from build123d import *

# Parameters (mm, degrees)
SKETCH1_R           = 4.064
BOSS_EXTRUDE1_DEPTH = 56.896
SKETCH2_R           = 15.24
BOSS_EXTRUDE2_DEPTH = 25.4
SKETCH3_R           = 17.501560838
BOSS_EXTRUDE3_DEPTH = 5.588


with BuildPart() as part:
    # Sketch1 → Boss-Extrude1 (new body)
    with BuildSketch(Plane(origin=(0, 0, 0), x_dir=(1, 0, 0), z_dir=(0, 1, 0))):
        with BuildLine():
            Line((-80.173724845, 32.537607562), (-20.229724845, 32.537607562))
            ThreePointArc((-20.229724845, 32.537607562), (-16.278412152, 30.900920256), (-14.641724845, 26.949607562))
            Line((-14.641724845, 26.949607562), (-14.641724845, -32.994392438))
            ThreePointArc((-14.641724845, -32.994392438), (-16.278412152, -36.945705131), (-20.229724845, -38.582392438))
            Line((-20.229724845, -38.582392438), (-80.173724845, -38.582392438))
            ThreePointArc((-80.173724845, -38.582392438), (-84.125037539, -36.945705131), (-85.761724845, -32.994392438))
            Line((-85.761724845, -32.994392438), (-85.761724845, 26.949607562))
            ThreePointArc((-85.761724845, 26.949607562), (-84.125037539, 30.900920256), (-80.173724845, 32.537607562))
        make_face()
        with Locations((-80.173724845, 26.949607562)):
            Circle(SKETCH1_R, mode=Mode.SUBTRACT)
        with Locations((-80.173724845, -32.994392438)):
            Circle(SKETCH1_R, mode=Mode.SUBTRACT)
        with Locations((-20.229724845, 26.949607562)):
            Circle(SKETCH1_R, mode=Mode.SUBTRACT)
        with Locations((-20.229724845, -32.994392438)):
            Circle(SKETCH1_R, mode=Mode.SUBTRACT)
    extrude(amount=BOSS_EXTRUDE1_DEPTH)

    # Sketch2 → Boss-Extrude2 (add)
    with BuildSketch(Plane.XZ):
        with Locations((-50.201724845, 3.022392438)):
            Circle(SKETCH2_R)
    extrude(amount=BOSS_EXTRUDE2_DEPTH)

    # Sketch3 → Boss-Extrude3 (add)
    with BuildSketch(Plane.XZ.offset(25.4)):
        with Locations((-50.201724845, 3.022392438)):
            Circle(SKETCH3_R)
    extrude(amount=BOSS_EXTRUDE3_DEPTH)


solid = part.part
Check sheet for the modelled part. Datum: model origin and axes. Units: mm. A direction names the side the tool comes from. Give positions to 0.01 mm unless a question says otherwise; leave off trailing zeros. Order: outer loops, then holes, each group sorted by start corner. A loop starts at its lowest first (then second) coordinate and runs counter-clockwise, first axis right, second up. Notation, with made-up numbers: (-10, 21.5) - (43, 21.5) arc R9 cw to (43, 30.5) - close; hole circle Ø5 at (-21, 44.5). An arc over 180 degrees is marked (long way). Answer as CSV lines item,"result".
1. Section check D-D (z = 14.5). Record the boundary of the cut face in (x, y), then the cut area to 3 significant figures.
Result sheet:
outline,"(-85.76, 0) - (-60.23, 0) - (-60.23, -25.4) - (-63.41, -25.4) - (-63.41, -30.99) - (-36.99, -30.99) - (-36.99, -25.4) - (-40.18, -25.4) - (-40.18, 0) - (-14.64, 0) - (-14.64, 56.9) - (-85.76, 56.9) - close"
area,"4,700 mm²"
2. Section check B-B (z = -24.5). Record the boundary of the cut face in (x, y).
Result sheet:
outline,"(-85.76, 0) - (-83.42, 0) - (-83.42, 56.9) - (-85.76, 56.9) - close; (-76.93, 0) - (-23.47, 0) - (-23.47, 56.9) - (-76.93, 56.9) - close; (-16.99, 0) - (-14.64, 0) - (-14.64, 56.9) - (-16.99, 56.9) - close"
3. Section check C-C (x = -19). Record the boundary of the cut face in (y, z).
Result sheet:
outline,"(0, -32.4) - (56.9, -32.4) - (56.9, -30.82) - (0, -30.82) - close; (0, -23.08) - (56.9, -23.08) - (56.9, 29.12) - (0, 29.12) - close; (0, 36.87) - (56.9, 36.87) - (56.9, 38.45) - (0, 38.45) - close"
4. Section check A-A (y = 5.5). Record the boundary of the cut face in (x, z), then the cut area to 3 significant figures.
Result sheet:
outline,"(-85.76, -26.95) arc R5.59 ccw to (-80.17, -32.54) - (-20.23, -32.54) arc R5.59 ccw to (-14.64, -26.95) - (-14.64, 32.99) arc R5.59 ccw to (-20.23, 38.58) - (-80.17, 38.58) arc R5.59 ccw to (-85.76, 32.99) - close; hole circle Ø8.13 at (-80.17, -26.95); hole circle Ø8.13 at (-80.17, 32.99); hole circle Ø8.13 at (-20.23, -26.95); hole circle Ø8.13 at (-20.23, 32.99)"
area,"4,820 mm²"
5. Scan lines: probe 1 along Z at (x, y) = (-80.5, 48.5); probe 2 along Z at (x, y) = (-80, 41.5); probe 3 along X at (y, z) = (15.5, -25). Record each from-to range of solid material in increasing order. Write a range as from..to.
Result sheet:
probe 1,"-32.53..-31, -22.9..28.94, 37.05..38.57"
probe 2,"-32.54..-31.01, -22.89..28.93, 37.05..38.58"
probe 3,"-85.76..-83.74, -76.61..-23.8, -16.66..-14.64"
6. Tool access check on faces 1 (the face through (-51, 28, -32.538)), 2 (the face through (-34.035, -28.155, -3.681)), 3 (the face through (-65.427, -12.522, 3.692)). Record the directions out of +Z, -Z, +X, -X, +Y, -Y that give a thin tool (end or side, any length) a straight path to the whole face; none if there is none.
Result sheet:
face 1,"-Z, +X, -X, +Y, -Y"
face 2,"-Y"
face 3,"none"
7. Mould release check, pull along Z, two halves, no side actions. Record for faces 4 (the face through (-16.32, 28.05, -30.94)), 5 (the face through (-85.762, 28, 3)), 6 (the face through (-18.354, 28.05, 36.6)): released by +Z, released by -Z, zero draft, split by the parting line, or undercut.
Result sheet:
face 4,"released by -Z"
face 5,"zero draft"
face 6,"undercut"
8. Go/stop test with flat-tipped pins: P1, Ø6.5, axis at x = -20.23, z = -26.95, coming from the -Y side; P2, Ø10.5, axis at x = -80.17, z = 32.99, coming from the -Y side. Record where each tip stops, or that it passes through.
Result sheet:
P1,"through"
P2,"y = 0"
